The model under review builds one solid part; all positions refer to its coordinate system, in mm. A direction names the side the tool comes from. Coordinates: 2 decimals unless noted, no trailing zeros. Write each loop counter-clockwise with the first axis right and the second up, starting at its lowest first coordinate (ties: lowest second). Pieces come first, ordered by that corner, then holes. Notation, with made-up numbers: (23.25, 9.25) - (37.25, 9.25) arc R21 ccw to (37.25, 43.25) - close; hole circle Ø3 at (79.25, -18.75). An arc over 180 degrees is marked (long way). Put each result on its own line as item: value. Start each with the question number.
Item 1: Consider section A-A on y = 31. Give the boundary of the cut face in (x, z), then the cut area to 3 significant figures.
Item 2: Mouldability with a two-part tool opening along Z and no side actions: class faces 3 (the face through (-2, 4, 3)), 4 (the face through (3.4, 0.5, -0.1)), 5 (the face through (-4.483, 53.209, 0.589)) as pulls with the +Z half, pulls with the -Z half, needs draft (parallel to the pull), parting line crosses it, or undercut.
Item 3: To check wall thickness, follow L1, parallel to Z at x = -3.25, y = 60; L2, parallel to Y at x = 0, z = 3.4; L3, parallel to Y at x = 0, z = 3.65. State the ranges of each line that lie inside material, in increasing order. Write a range as [from, to].
Item 4: Consider section B-B on y = 73.5. Give the boundary of the cut face in (x, z), then the cut area to 3 significant figures.
Item 5: For pin 1 (1.2 mm diameter, centred on x = -1.5, y = 3.5, fed in from +Z); pin 2 (4 mm diameter, centred on y = 27, z = 2, fed in from -X); pin 3 (6 mm diameter, centred on x = -3, z = 3, fed in from +Y), all flat-tipped, find the tip position at first contact; note any pin that passes through.
Item 6: Machinability: for faces 1 (the face through (-1, 7, 0)), 2 (the face through (-2.24, 0.77, 3.73)), which of the approach directions +Z, -Z, +X, -X, +Y, -Y give a long, thin tool a straight path to every point of the face, cutting with its end or side? Answer none if there is none.
```python
from build123d import *

# Parameters (mm, degrees)
CUT_EXTRUDE1_DEPTH      = 91.700053892
CUT_EXTRUDE1_DEPTH_BACK = 91.700053892
CUT_EXTRUDE2_DEPTH      = 91.700053903
CUT_EXTRUDE2_DEPTH_BACK = 91.700053903
SKETCH7_R               = 0.5
CUT_EXTRUDE3_DEPTH      = 6.5


with BuildPart() as part:
    # Sketch2 → Revolve1 (revolve)
    with BuildSketch(Plane.XY, mode=Mode.PRIVATE) as revolve1_sk:
        with BuildLine():
            Line((0, 0), (5, 0))
            Line((5, 0), (5, 19.05))
            Line((5, 19.05), (4.056413105, 86.424))
            ThreePointArc((4.056413105, 86.424), (2.848441999, 89.255803453), (0, 90.424))
            Line((0, 90.424), (0, 0))
        make_face()
    revolve(revolve1_sk.sketch.rotate(Axis((0, 0, 0), (0, 1, 0)), 90), axis=Axis((0, 0, 0), (0, 1, 0)))

    # Sketch6 → Cut-Extrude1 (cut, two sides: drawn at the far end of the back side and taken through both)
    with BuildSketch(Plane.XY.offset(-CUT_EXTRUDE1_DEPTH_BACK)):
        with BuildLine():
            Line((-4, 3.5), (-4, 7))
            Line((-4, 7), (-5, 8))
            Line((-5, 8), (-5, 0))
            Line((-5, 0), (5, 0))
            Line((5, 0), (5, 0.5))
            Line((5, 0.5), (-1, 0.5))
            ThreePointArc((-1, 0.5), (-3.121320344, 1.378679656), (-4, 3.5))
        make_face()
    extrude(amount=CUT_EXTRUDE1_DEPTH + CUT_EXTRUDE1_DEPTH_BACK, mode=Mode.SUBTRACT)

    # Sketch7 → Cut-Extrude2 (cut, two sides: drawn at the far end of the back side and taken through both)
    with BuildSketch(Plane.XY.offset(-CUT_EXTRUDE2_DEPTH_BACK)):
        with Locations((0, 4.7625)):
            Circle(SKETCH7_R)
    extrude(amount=CUT_EXTRUDE2_DEPTH + CUT_EXTRUDE2_DEPTH_BACK, mode=Mode.SUBTRACT)

    # Sketch8 → Cut-Extrude3 (cut)
    with BuildSketch(Plane.XZ.offset(-0.5)):
        with BuildLine():
            Line((0, 3), (-5, 3))
            Line((-5, 3), (-5, -3))
            Line((-5, -3), (0, -3))
            ThreePointArc((0, -3), (3, 0), (0, 3))
        make_face()
    extrude(amount=-CUT_EXTRUDE3_DEPTH, mode=Mode.SUBTRACT)


solid = part.part
```
Report:
1. outline: circle Ø9.67 at (0, 0)
1. area: 73.4 mm²
2. face 3: undercut
2. face 4: needs draft
2. face 5: parting line crosses it
3. L1: [-3.01, 3.01]
3. L2: [0.5, 4.26], [5.26, 88.58]
3. L3: [0.5, 4.26], [5.26, 88.14]
4. outline: circle Ø8.47 at (0, 0)
4. area: 56.4 mm²
5. pin 1: z = 4.92
5. pin 2: x = -4.9
5. pin 3: y = 90.23
6. face 1: -X, -Y
6. face 2: +Z, -Z, -X, -Y
